The model under review builds one solid part; all positions refer to its coordinate system, in mm. A direction names the side the tool comes from. Coordinates: 2 decimals unless noted, no trailing zeros. Write each loop counter-clockwise with the first axis right and the second up, starting at its lowest first coordinate (ties: lowest second). Pieces come first, ordered by that corner, then holes.
```python
from build123d import *

# Parameters (mm, degrees)
F0_W     = 300
F0_H     = 250
F1_DEPTH = 15
F2_R     = 95.409832
F3_DEPTH = 12
F4_R     = 12.5
F5_DEPTH = 15.001
F6_W     = 220
F6_H     = 3
F7_DEPTH = 40


with BuildPart() as f1:
    # F0 (on Top) → F1 (new body)
    with BuildSketch(Plane.XY):
        Rectangle(F0_W, F0_H)
    extrude(amount=F1_DEPTH)

    # F2 (on face) → F3 (cut)
    with BuildSketch(Plane.XY.offset(15)):
        Circle(F2_R)
    extrude(amount=-F3_DEPTH, mode=Mode.SUBTRACT)

    # F4 (on face) → F5 (cut, through all)
    with BuildSketch(Plane.XY.offset(15)):
        Circle(F4_R)
    extrude(amount=-F5_DEPTH, mode=Mode.SUBTRACT)

    # F6 (on face) → F7 (join)
    with BuildSketch(Plane.XY.offset(15)):
        with Locations((0, 123.5)):
            Rectangle(F6_W, F6_H)
        with Locations((0, -123.5)):
            Rectangle(F6_W, F6_H)
    extrude(amount=F7_DEPTH)


solid = f1.part
```
Item 1: Take a section at D-D, the plane y = -105.5. Write out the cut boundary in (x, z), plus the area to 3 significant figures.
Solved:
outline: (-150, 0) - (150, 0) - (150, 15) - (-150, 15) - close
area: 4,500 mm2
Item 2: For pin 1 (0.9 mm diameter, centred on y = -123.5, z = 34.5, fed in from -X); pin 2 (15 mm diameter, centred on x = 0, y = 0, fed in from +Z); pin 3 (0.9 mm diameter, centred on y = -124, z = 33, fed in from +X); pin 4 (6 mm diameter, centred on x = -30, y = -90, fed in from +Z), all flat-tipped, find the tip position at first contact; note any pin that passes through.
Solved:
pin 1: stops at x = -110
pin 2: passes through
pin 3: stops at x = 110
pin 4: stops at z = 15
Item 3: Take a section at C-C, the plane x = -104. Write out the cut boundary in (y, z).
Solved:
outline: (-125, 0) - (125, 0) - (125, 55) - (122, 55) - (122, 15) - (-122, 15) - (-122, 55) - (-125, 55) - close
Item 4: Mouldability with a two-part tool opening along X and no side actions: class faces 4 (the face through (-1, -20, 3)), 5 (the face through (-102, 2, 15)), 6 (the face through (-150, -2, 7)) as pulls with the +X half, pulls with the -X half, needs draft (parallel to the pull), parting line crosses it, or undercut.
Solved:
face 4: undercut
face 5: needs draft
face 6: pulls with the -X half
Item 5: Take a section at A-A, the plane z = 22.5. Write out the cut boundary in (x, y).
Solved:
outline: (-110, -125) - (110, -125) - (110, -122) - (-110, -122) - close; (-110, 122) - (110, 122) - (110, 125) - (-110, 125) - close
Item 6: To check wall thickness, follow line 1 along Y through (x, z) = (69.5, 27.5); line 2 along Y through (x, z) = (0, 1); line 3 along Z through (x, y) = (16, 14). State the ranges of each line that lie inside material, in increasing order.
Solved:
line 1: y = -125 to -122, 122 to 125
line 2: y = -125 to -12.5, 12.5 to 125
line 3: z = 0 to 3
Item 7: Machinability: for faces 1 (the face through (-2, -122, 35)), 2 (the face through (-20.68, -93.14, 9.08)), 3 (the face through (150, -2, 7)), which of the approach directions +Z, -Z, +X, -X, +Y, -Y give a long, thin tool a straight path to every point of the face, cutting with its end or side? Answer none if there is none.
Solved:
face 1: +Z, +X, -X
face 2: +Z
face 3: +Z, -Z, +X, +Y, -Y
Item 8: Take a section at B-B, the plane y = 0. Write out the cut boundary in (x, z), plus the area to 3 significant figures.
Solved:
outline: (-150, 0) - (-12.5, 0) - (-12.5, 3) - (-95.41, 3) - (-95.41, 15) - (-150, 15) - close; (12.5, 0) - (150, 0) - (150, 15) - (95.41, 15) - (95.41, 3) - (12.5, 3) - close
area: 2,140 mm2
